Here's how the part is built. I have some questions about the finished solid (model axes, mm). A direction names the side the tool comes from. Round coordinates to 2 decimals unless told otherwise and drop trailing zeros. Write each loop counter-clockwise with the first axis right and the second up, starting at its lowest first coordinate (ties: lowest second). Pieces come first, ordered by that corner, then holes. Notation, with made-up numbers: (21, 85) - (55, 85) arc R24 ccw to (55, 116) - close; hole circle Ø1 at (31, 3.5). An arc over 180 degrees is marked (long way). Write item = value, one per line. Start each with the question number.
Item 1: For P1, Ø1.5, axis at x = 11, z = -24, coming from the -Y side; P2, Ø8, axis at y = -176.5, z = -7.5, coming from the +X side; P3, Ø10, axis at y = -128.5, z = -44.5, coming from the -X side, each with a flat end and sliding along its axis, tell me the tip position at first contact or that it passes through.
Item 2: If we section it at A-A (x = 19): Please give me the cut outline in (y, z).
Item 3: If we section it at B-B (y = -324): Please give me the cut outline in (x, z).
Item 4: Thinking about a two-plate mould opening in Z: for faces 3 (the face through (19.35, -192.27, -34.51)), 4 (the face through (4.358, -192.27, -35.49)), 5 (the face through (11.688, -4.237, 34.51)), which applies, pulls with the +Z half, pulls with the -Z half, needs draft (parallel to the pull), parting line crosses it, or undercut?
Item 5: If I drill on line 1 along X through (y, z) = (-327, 0.5); line 2 along X through (y, z) = (-310, -27.5); line 3 along Y through (x, z) = (4.75, -10), over which ranges is the centre line in solid material (lowest first)? Write a range as [from, to].
Item 6: If we section it at C-C (z = 7): Please give me the cut outline in (x, y), and give its area (3 significant figures).
Item 7: If we section it at D-D (z = 24.5): Please give me the cut outline in (x, y).
Item 8: Which directions (+Z, -Z, +X, -X, +Y, -Y) give clear straight access to the entire face, cutting with the end or side of a thin tool? Please do faces 1 (the face through (19.35, -192.27, 34.51)), 2 (the face through (11.688, -385.642, 35.49)).
```python
from build123d import *

# Parameters (mm, degrees)
F1_DEPTH = 460
F3_DEPTH = 37.493171


with BuildPart() as f1:
    # F0 (on Front) → F1 (new body)
    with BuildSketch(Plane.XZ):
        Polygon((0, 0), (15.112647, 0), (37.492171, 182.266595), (22.603979, 184.094635), align=None)
    extrude(amount=F1_DEPTH)

    # F2 (on Right) → F3 (intersect, through all)
    with BuildSketch(Plane.YZ):
        Polygon((-390, 0), (0, 0), (-8.594919, 70), (-381.405081, 70), align=None)
    extrude(amount=F3_DEPTH, mode=Mode.INTERSECT)

    # F4: F1 across face


with BuildPart() as f1_1:
    add(f1.part)
    add(f1.part.mirror(Plane(origin=(7.556324, -195, 0), x_dir=(1, 0, 0), z_dir=(0, 0, -1))))


solid = f1_1.part
```
Reply:
q1.P1 = -387.15
q1.P2 = 16.52
q1.P3 = 4.85
q2.outline = (-386.11, -31.66) - (-381.41, -70) - (-8.59, -70) - (-3.89, -31.66) - close; (-386.11, 31.66) - (-3.89, 31.66) - (-8.59, 70) - (-381.41, 70) - close
q3.outline = (0, 0) - (8.59, -70) - (23.71, -70) - (15.11, 0) - (23.71, 70) - (8.59, 70) - close
q4.face_3 = undercut
q4.face_4 = pulls with the -Z half
q4.face_5 = pulls with the +Z half
q5.line_1 = [0.06, 15.17]
q5.line_2 = [3.38, 18.49]
q5.line_3 = [-388.77, -1.23]
q6.outline = (0.86, -389.14) - (15.97, -389.14) - (15.97, -0.86) - (0.86, -0.86) - close
q6.area = 5,870 mm2
q7.outline = (3.01, -386.99) - (18.12, -386.99) - (18.12, -3.01) - (3.01, -3.01) - close
q8.face_1 = +X, +Y, -Y
q8.face_2 = +Z, +X, -X, -Y
